Drawing for the job (mm, zero at the part's lowest x, y, z). Coordinates: 2 decimals unless noted, no trailing zeros. Write each loop counter-clockwise with the first axis right and the second up, starting at its lowest first coordinate (ties: lowest second). Pieces come first, ordered by that corner, then holes. Notation, with made-up numbers: (-17.5, -4.75) - (34.5, -4.75) arc R14 ccw to (34.5, 22.25) - close; hole circle Ø10 at (6, 47.25). An arc over 180 degrees is marked (long way). Write each question's results on one line, items separated by ' | '.
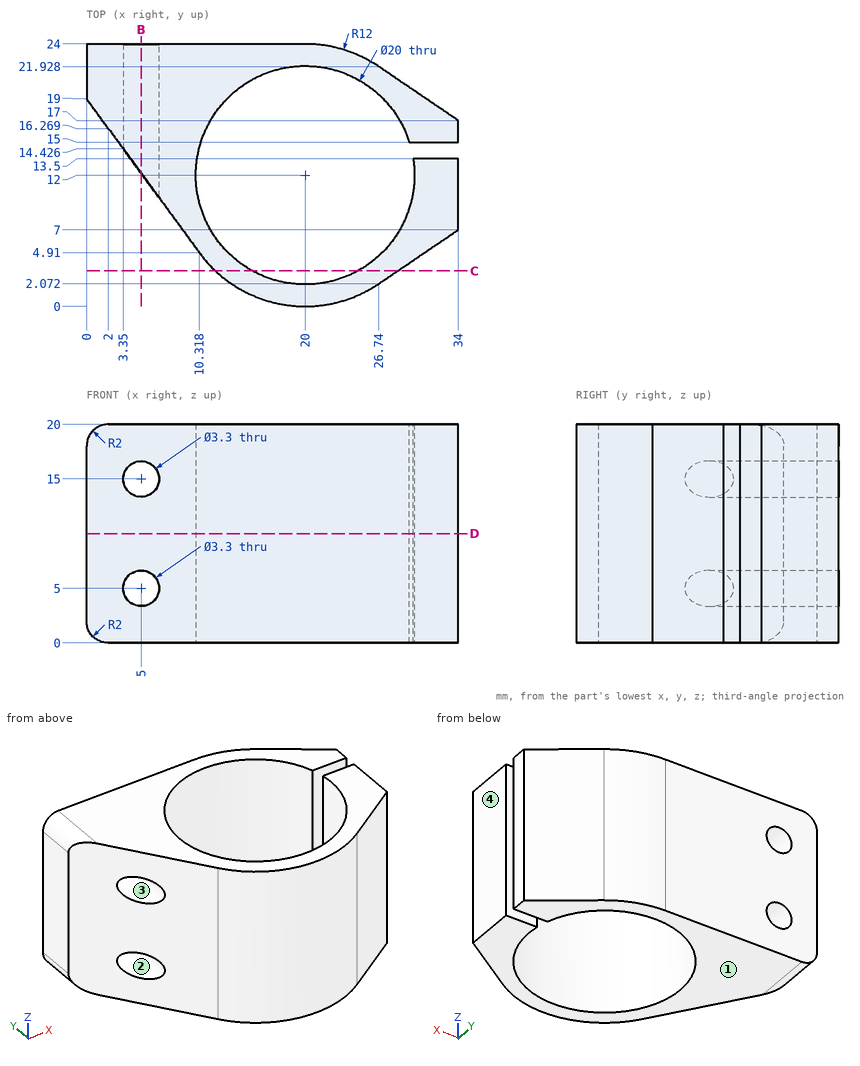
(1) Flat gauge pins, fed straight in: P1, Ø1.2, axis at x = 32, z = 6, coming from the +Y side (1 decimal); P2, Ø5, axis at y = 15.5, z = 17, coming from the -X side; P3, Ø3.5, axis at x = 33, z = 5.5, coming from the -Y side; P4, Ø3, axis at x = 5, z = 5, coming from the -Y side. Where does each tip first touch, or does it go through?
Return value:
P1: stops at y = 18.8 | P2: stops at x = 0.73 | P3: stops at y = 5.13 | P4: passes through
(2) Wall check: line 1 (Z direction, x = 5, y = 20.5); line 2 (Y direction, x = 20, z = 13); line 3 (X direction, y = 19.5, z = 4) (1 decimal). Give the ranges that are in metal, low to high. Write a range as from..to.
Return value:
line 1: z = 0..3.35, 6.65..13.35, 16.65..20 | line 2: y = 0..2, 22..24 | line 3: x = 0..3.7, 6.3..13.4, 26.6..30.3
(3) Saw through at C-C on y = 3.25. Write the cut outline in (x, z) (1 decimal).
Return value:
outline: (11.8, 0) - (15.2, 0) - (15.2, 20) - (11.8, 20) - close; (24.8, 0) - (28.5, 0) - (28.5, 20) - (24.8, 20) - close
(4) Two-plate mould, pull along Z, no slides. Class the marked faces 1, 2, 3 and 4: released by +Z, released by -Z, zero draft, split by the parting line, or undercut.
Return value:
face 1: released by -Z | face 2: undercut | face 3: undercut | face 4: zero draft
(5) Saw through at D-D on z = 10. Write the cut outline in (x, y), then the cut area to 3 significant figures.
Return value:
outline: (0, 19) - (10.32, 4.91) arc R12 ccw to (26.74, 2.07) - (34, 7) - (34, 13.5) - (29.89, 13.5) arc R10 cw (long way) to (29.54, 15) - (34, 15) - (34, 17) - (26.74, 21.93) arc R12 ccw to (20, 24) - (0, 24) - close | area: 283 mm^2
(6) Saw through at B-B on x = 5. Write the cut outline in (y, z).
Return value:
outline: (12.17, 0) - (24, 0) - (24, 3.35) - (12.17, 3.35) - close; (12.17, 6.65) - (24, 6.65) - (24, 13.35) - (12.17, 13.35) - close; (12.17, 16.65) - (24, 16.65) - (24, 20) - (12.17, 20) - close
